For this review, take the finished solid that the model builds, in its own axes (mm). Face numbers are marked on the shaded views. A direction names the side the tool comes from. Coordinates: 2 decimals unless noted, no trailing zeros. Order: outer loops, then holes, each group sorted by start corner. A loop starts at its lowest first (then second) coordinate and runs counter-clockwise, first axis right, second up. Notation, with made-up numbers: (41.25, 15.25) -> (99.25, 15.25) arc R23 ccw to (99.25, 26.25) -> close; hole circle Ø5 at (31.25, 21). An arc over 180 degrees is marked (long way). Write item = value, one per line. Start each with the question number.
1) Consider section B-B on z = 0. Give the boundary of the cut face in (x, y).
2) Draft analysis for pull direction X (two halves, no side actions). For the marked faces 3, 4 and 5, state which applies: +X half, -X half, draft (parallel to the pull), parting line (faces both ways), or undercut.
3) Consider section A-A on x = 0. Give the boundary of the cut face in (y, z).
4) Consider section C-C on x = 5.5. Give the boundary of the cut face in (y, z), and give its area (3 significant figures).
5) Machinability: for the marked faces 1 and 2, which of the approach directions +Z, -Z, +X, -X, +Y, -Y give a long, thin tool a straight path to every point of the face, cutting with its end or side? Answer none if there is none.
6) Wall thickness on probe 1 along X at (y, z) = (50, -8.25); probe 2 along Z at (x, y) = (-6.25, 43): over which ranges is each line inside the solid? List them lowest first. Write a range as [from, to].
7) Insertion check: pin 1 Ø6 at (x, y) = (3, 18) entering from +Z; pin 2 Ø4 at (x, y) = (0.5, 60.5) entering from -Z; pin 3 Ø1.8 at (y, z) = (70.5, 1.5) entering from +X. Each pin has a flat end and moves straight along its axis. Give the tip position at first contact, or say it passes through.
8) Consider section D-D on z = -5.75. Give the boundary of the cut face in (x, y).
from build123d import *

# Parameters (mm, degrees)
F_2020_SKETCH_R     = 3
BOSS_EXTRUDE1_DEPTH = 100


with BuildPart() as part:
    # 2020 sketch → Boss-Extrude1 (new body)
    with BuildSketch(Plane(origin=(0, 0, 0), x_dir=(1, 0, 0), z_dir=(0, 1, 0))):
        Polygon((-4, 10), (-4, 8), (-7, 8), (-3, 4), (3, 4), (7, 8), (4, 8), (4, 10), (10, 10), (10, 4), (8, 4), (8, 7), (4, 3), (4, -3), (8, -7), (8, -4), (10, -4), (10, -10), (4, -10), (4, -8), (7, -8), (3, -4), (-3, -4), (-7, -8), (-4, -8), (-4, -10), (-10, -10), (-10, -4), (-8, -4), (-8, -7), (-4, -3), (-4, 3), (-8, 7), (-8, 4), (-10, 4), (-10, 10), align=None)
        with Locations(Location((0, 0, 0), (0, 0, 270))):
            Circle(F_2020_SKETCH_R, mode=Mode.SUBTRACT)
    extrude(amount=BOSS_EXTRUDE1_DEPTH)


solid = part.part
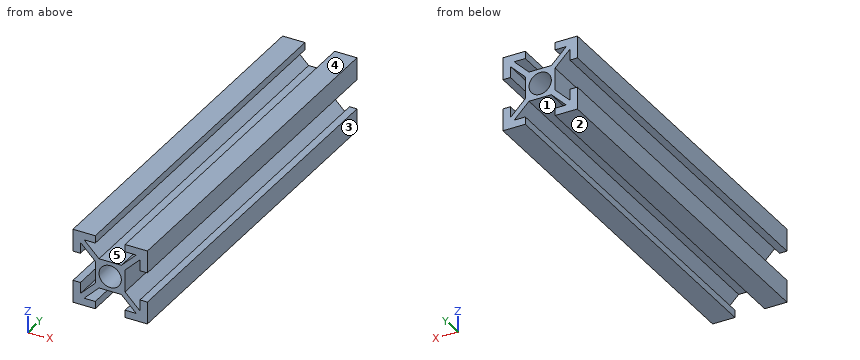
Answer sheet:
q1.outline = (-4, 0) -> (-3, 0) -> (-3, 100) -> (-4, 100) -> close; (3, 0) -> (4, 0) -> (4, 100) -> (3, 100) -> close
q2.face_3 = +X half
q2.face_4 = draft
q2.face_5 = undercut
q3.outline = (0, -4) -> (100, -4) -> (100, -3) -> (0, -3) -> close; (0, 3) -> (100, 3) -> (100, 4) -> (0, 4) -> close
q4.outline = (0, -10) -> (100, -10) -> (100, -8) -> (0, -8) -> close; (0, -6.5) -> (100, -6.5) -> (100, -4.5) -> (0, -4.5) -> close; (0, 4.5) -> (100, 4.5) -> (100, 6.5) -> (0, 6.5) -> close; (0, 8) -> (100, 8) -> (100, 10) -> (0, 10) -> close
q4.area = 800 mm2
q5.face_1 = -Z, +Y, -Y
q5.face_2 = -Z, +X, -X, +Y, -Y
q6.probe_1 = [-10, -4], [4, 10]
q6.probe_2 = [-10, -8], [-7.25, -5.25], [5.25, 7.25], [8, 10]
q7.pin_1 = 10
q7.pin_2 = -4
q7.pin_3 = 4
q8.outline = (-10, 0) -> (-8, 0) -> (-8, 100) -> (-10, 100) -> close; (-6.75, 0) -> (-4.75, 0) -> (-4.75, 100) -> (-6.75, 100) -> close; (4.75, 0) -> (6.75, 0) -> (6.75, 100) -> (4.75, 100) -> close; (8, 0) -> (10, 0) -> (10, 100) -> (8, 100) -> close
